For this review, take the finished solid that the model builds, in its own axes (mm). Face numbers are marked on the shaded views. A direction names the side the tool comes from. Coordinates: 2 decimals unless noted, no trailing zeros. Write each loop counter-clockwise with the first axis right and the second up, starting at its lowest first coordinate (ties: lowest second). Pieces come first, ordered by that corner, then holes. Notation, with made-up numbers: (88.5, 31.5) - (135.5, 31.5) arc R13 cw to (135.5, 43.5) - close; hole circle Ø3 at (-24, -13.5). An arc over 180 degrees is marked (long way). Write each question's results on one line, items separated by ' | '.
from build123d import *

# Parameters (mm, degrees)
SKETCH1_R           = 17.5
BOSS_EXTRUDE1_DEPTH = 55
SKETCH2_R           = 9.525
CUT_EXTRUDE1_DEPTH  = 23
CUT_EXTRUDE2_REACH  = 42.454
SKETCH5_R           = 6
CUT_EXTRUDE3_DEPTH  = 23


with BuildPart() as part:
    # Sketch1 → Boss-Extrude1 (new body)
    with BuildSketch(Plane(origin=(0, 0, 0), x_dir=(1, 0, 0), z_dir=(0, 1, 0))):
        with Locations(Location((0, 0, 0), (0, 0, 270))):
            Circle(SKETCH1_R)
    extrude(amount=BOSS_EXTRUDE1_DEPTH)

    # Sketch2 → Cut-Extrude1 (cut)
    with BuildSketch(Plane(origin=(0, 55, 0), x_dir=(1, 0, 0), z_dir=(0, 1, 0))):
        with Locations(Location((0, 0, 0), (0, 0, 270))):
            Circle(SKETCH2_R)
    extrude(amount=-CUT_EXTRUDE1_DEPTH, mode=Mode.SUBTRACT)

    # Sketch3 → Cut-Extrude2 (cut, up to next)
    with BuildSketch(Plane(origin=(0, 32, 0), x_dir=(1, 0, 0), z_dir=(0, 1, 0)), mode=Mode.PRIVATE) as cut_extrude2_sk1:
        Polygon((9.525, 2.37), (11.625, 2.37), (11.625, -2.366924295), (6.895, -2.366924295), (6.895, 2.37), align=None)
    cut_extrude2_tool1 = extrude(cut_extrude2_sk1.sketch, amount=CUT_EXTRUDE2_REACH, mode=Mode.PRIVATE) & part.part
    add(cut_extrude2_tool1.solids().sort_by_distance((9.26, 32, -0.001538))[0], mode=Mode.SUBTRACT)

    # Sketch5 → Cut-Extrude3 (cut)
    with BuildSketch(Plane(origin=(0, 0, 0), x_dir=(-1, 0, 0), z_dir=(0, -1, 0))):
        with Locations(Location((0, 0, 0), (0, 0, 90))):
            Circle(SKETCH5_R)
    extrude(amount=-CUT_EXTRUDE3_DEPTH, mode=Mode.SUBTRACT)


solid = part.part
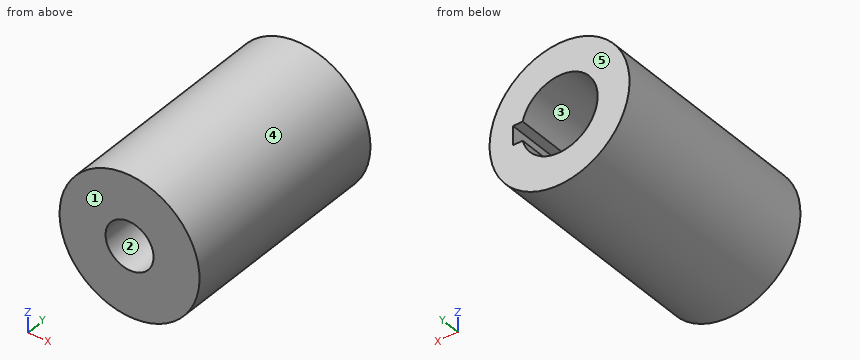
Q1. Take a section at C-C on z = 0. State the section outline as (x, y) points (3 decimals), plus the area to 3 significant figures.
Results found:
outline: (-17.5, 0) - (-6, 0) - (-6, 23) - (6, 23) - (6, 0) - (17.5, 0) - (17.5, 55) - (11.625, 55) - (11.625, 32) - (-9.525, 32) - (-9.525, 55) - (-17.5, 55) - close | area: 1,160 mm2
Q2. For the marked faces 1 and 2, list the 3-axis set-ups (+Z, -Z, +X, -X, +Y, -Y) from which the entire face can be reached by the end or side of a thin tool; tool diameter is ignored.
Results found:
face 1: +Z, -Z, +X, -X, -Y | face 2: -Y
Q3. For pin 1 (1 mm diameter, centred on x = -9.5, y = 24, fed in from -Z); pin 2 (6 mm diameter, centred on x = -8, y = 15.5, fed in from -Z); pin 3 (12 mm diameter, centred on y = 38, z = -6.5, fed in from +X), all flat-tipped, find the tip position at first contact; note any pin that passes through.
Results found:
pin 1: z = -15.01 | pin 2: z = -16.77 | pin 3: x = 17.49
Q4. Mouldability with a two-part tool opening along X and no side actions: class the marked faces 3, 4 and 5 as pulls with the +X half, pulls with the -X half, needs draft (parallel to the pull), parting line crosses it, or undercut.
Results found:
face 3: undercut | face 4: parting line crosses it | face 5: needs draft
Q5. Wall thickness on line 1 along X through (y, z) = (15, 0); line 2 along X through (y, z) = (38, 0) (3 decimals); line 3 along Y through (x, z) = (-8.5, -2.5): over which ranges is each line inside the solid? List them lowest first. Write a range as from..to.
Results found:
line 1: -17.5..-6, 6..17.5 | line 2: -17.5..-9.525, 11.625..17.5 | line 3: 0..32
Q6. Take a section at A-A on y = 47.5. State the section outline as (x, z) points (3 decimals), plus the area to 3 significant figures.
Results found:
outline: circle Ø35 at (0, 0); hole (9.225, -2.37) - (11.625, -2.37) - (11.625, 2.367) - (9.226, 2.367) arc R9.525 ccw (long way) to start | area: 667 mm2
Q7. Take a section at D-D on y = 21.5. State the section outline as (x, z) points.
Results found:
outline: circle Ø35 at (0, 0); hole circle Ø12 at (0, 0)
Q8. Take a section at B-B on x = 0. State the section outline as (y, z) points (3 decimals), plus the area to 3 significant figures.
Results found:
outline: (0, -17.5) - (55, -17.5) - (55, -9.525) - (32, -9.525) - (32, 9.525) - (55, 9.525) - (55, 17.5) - (0, 17.5) - (0, 6) - (23, 6) - (23, -6) - (0, -6) - close | area: 1,210 mm2
